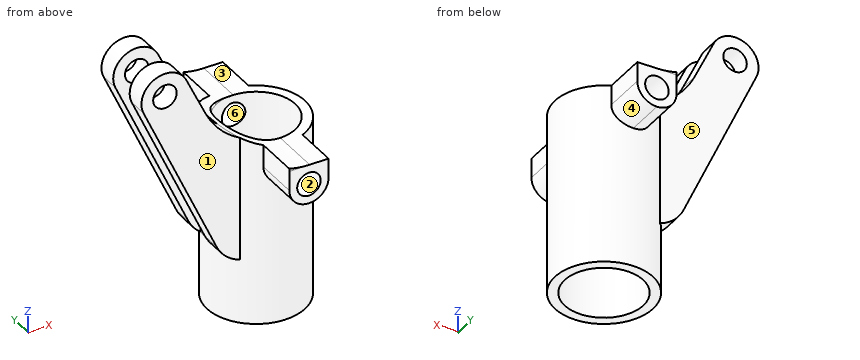
```python
from build123d import *

# Parameters (mm, degrees)
CROQUIS1_R                   = 6.25
CROQUIS1_R_2                 = 5
SALIENTE_EXTRUIR1_DEPTH      = 15
SALIENTE_EXTRUIR2_REACH      = 25.881
SALIENTE_EXTRUIR2_END_RADIUS = 6.25
CROQUIS2_W                   = 5
CROQUIS2_H                   = 5
SALIENTE_EXTRUIR3_REACH      = 29.755
SALIENTE_EXTRUIR3_END_RADIUS = 6.25
CROQUIS3_W                   = 5
CROQUIS3_H                   = 5
CORTAR_EXTRUIR1_REACH        = 29.755
CROQUIS4_R                   = 1.5
REDONDEO1_R                  = 2.5
CROQUIS5_R                   = 1.5
SALIENTE_EXTRUIR4_DEPTH      = 2.5
SALIENTE_EXTRUIR5_REACH      = 34.452
CROQUIS6_W                   = 15
CROQUIS6_H                   = 2.5
CROQUIS7_R                   = 1.5
SALIENTE_EXTRUIR6_DEPTH      = 2.5
SALIENTE_EXTRUIR7_REACH      = 34.452
SALIENTE_EXTRUIR7_END_RADIUS = 6.25
CROQUIS8_W                   = 15
CROQUIS8_H                   = 2.5
REDONDEO2_R                  = 5
REDONDEO4_R                  = 10
SALIENTE_EXTRUIR9_REACH      = 43.224
CROQUIS10_R                  = 6.25
CROQUIS10_R_2                = 5


# Some blends are built 0.0001 mm under size
with BuildPart() as part:
    # Croquis1 → Saliente-Extruir1 (new body)
    with BuildSketch(Plane.XY):
        Circle(CROQUIS1_R)
        Circle(CROQUIS1_R_2, mode=Mode.SUBTRACT)
    extrude(amount=SALIENTE_EXTRUIR1_DEPTH)

    # Saliente-Extruir2: up to this cylinder (the profile starts outside it)
    saliente_extruir2_end = Plane(origin=(0, 0, 12.5), z_dir=(0, 0, -1)) * Cylinder(SALIENTE_EXTRUIR2_END_RADIUS, 65.262, mode=Mode.PRIVATE)
    # Croquis2 → Saliente-Extruir2 (add, up to the surface)
    with BuildSketch(Plane(origin=(0, 11.25, 0), x_dir=(1, 0, 0), z_dir=(0, 1, 0)), mode=Mode.PRIVATE) as saliente_extruir2_sk1:
        with Locations((0, -12.5)):
            Rectangle(CROQUIS2_W, CROQUIS2_H)
    saliente_extruir2_tool1 = extrude(saliente_extruir2_sk1.sketch, amount=-SALIENTE_EXTRUIR2_REACH, mode=Mode.PRIVATE) - saliente_extruir2_end
    add(saliente_extruir2_tool1.solids().sort_by_distance((0, 11.25, 12.5))[0])

    # Saliente-Extruir3: up to this cylinder (the profile starts outside it)
    saliente_extruir3_end = Plane(origin=(0, 0, 12.5), z_dir=(0, 0, -1)) * Cylinder(SALIENTE_EXTRUIR3_END_RADIUS, 73.01, mode=Mode.PRIVATE)
    # Croquis3 → Saliente-Extruir3 (add, up to the surface)
    with BuildSketch(Plane(origin=(0, -11.25, 0), x_dir=(1, 0, 0), z_dir=(0, 1, 0)), mode=Mode.PRIVATE) as saliente_extruir3_sk1:
        with Locations((0, -12.5)):
            Rectangle(CROQUIS3_W, CROQUIS3_H)
    saliente_extruir3_tool1 = extrude(saliente_extruir3_sk1.sketch, amount=SALIENTE_EXTRUIR3_REACH, mode=Mode.PRIVATE) - saliente_extruir3_end
    add(saliente_extruir3_tool1.solids().sort_by_distance((0, -11.25, 12.5))[0])

    # Cortar-Extruir1: up to this face of the body (flat: up to its plane)
    cortar_extruir1_end = Plane(part.part.faces().sort_by_distance((0, -11.25, 12.5))[0])
    # Croquis4 → Cortar-Extruir1 (cut, up to the picked face)
    with BuildSketch(Plane(origin=(0, 11.25, 0), x_dir=(1, 0, 0), z_dir=(0, 1, 0)), mode=Mode.PRIVATE) as cortar_extruir1_sk1:
        with Locations(Location((0, -12.5, 0), (0, 0, 270))):
            Circle(CROQUIS4_R)
    cortar_extruir1_tool1 = split(extrude(cortar_extruir1_sk1.sketch, amount=-CORTAR_EXTRUIR1_REACH, mode=Mode.PRIVATE), bisect_by=cortar_extruir1_end, keep=Keep.BOTH, mode=Mode.PRIVATE)
    add(cortar_extruir1_tool1.solids().sort_by(Axis((0, 11.25, 12.5), (0, -1, 0)))[0], mode=Mode.SUBTRACT)

    # Redondeo1
    redondeo1_edges = [part.edges().sort_by_distance(p)[0] for p in [
        (-2.5, -8.489109809, 10),
        (2.5, -8.489109809, 10),
        (-2.5, 8.489109809, 10),
        (2.5, 8.489109809, 10),
    ]]
    fillet(redondeo1_edges, radius=REDONDEO1_R - 0.0001)  # a hair under: the kernel refuses the full size

    # Croquis6 → Saliente-Extruir5 (add, up to next)
    with BuildSketch(Plane(origin=(-6.25, 0, 0), x_dir=(0, 0, -1), z_dir=(1, 0, 0)), mode=Mode.PRIVATE) as saliente_extruir5_sk1:
        with Locations((-7.5, -3)):
            Rectangle(CROQUIS6_W, CROQUIS6_H)
    saliente_extruir5_tool1 = extrude(saliente_extruir5_sk1.sketch, amount=SALIENTE_EXTRUIR5_REACH, mode=Mode.PRIVATE) - part.part


with BuildPart() as body_2:
    # Croquis5 → Saliente-Extruir4 (new body)
    with BuildSketch(Plane(origin=(0, -4.25, 0), x_dir=(1, 0, 0), z_dir=(0, 1, 0))):
        with BuildLine():
            Line((-6.25, -15), (-11.445879417, -26.033157432))
            ThreePointArc((-11.445879417, -26.033157432), (-15.41753329, -27.478700895), (-16.893124871, -23.518112569))
            Line((-16.893124871, -23.518112569), (-6.25, 0))
            Line((-6.25, 0), (-6.25, -15))
        make_face()
        with Locations(Location((-14.159974768, -24.755, 0), (0, 0, 270))):
            Circle(CROQUIS5_R, mode=Mode.SUBTRACT)
    extrude(amount=SALIENTE_EXTRUIR4_DEPTH)


with BuildPart() as part_1:
    add(part.part)

    add(body_2.part)  # Saliente-Extruir5 merges body 2
    add(saliente_extruir5_tool1.solids().sort_by_distance((-6.25, -3, 7.5))[0])



with BuildPart() as body_2_2:
    # Croquis7 → Saliente-Extruir6 (new body)
    with BuildSketch(Plane(origin=(0, 4.25, 0), x_dir=(1, 0, 0), z_dir=(0, 1, 0))):
        with BuildLine():
            Line((-11.445879417, -26.033157432), (-6.25, -15))
            Line((-6.25, -15), (-6.25, 0))
            Line((-6.25, 0), (-16.893124871, -23.518112569))
            ThreePointArc((-16.893124871, -23.518112569), (-15.41753329, -27.478700895), (-11.445879417, -26.033157432))
        make_face()
        with Locations(Location((-14.159974768, -24.755, 0), (0, 0, 270))):
            Circle(CROQUIS7_R, mode=Mode.SUBTRACT)
    extrude(amount=-SALIENTE_EXTRUIR6_DEPTH)


with BuildPart() as part_2:
    add(part_1.part)

    add(body_2_2.part)  # Saliente-Extruir7 merges body 2 2
    # Saliente-Extruir7: up to this cylinder (the profile starts outside it)
    saliente_extruir7_end = Plane(origin=(0, 0, 7.5), z_dir=(0, 0, -1)) * Cylinder(SALIENTE_EXTRUIR7_END_RADIUS, 82.404, mode=Mode.PRIVATE)
    # Croquis8 → Saliente-Extruir7 (add, up to the surface)
    with BuildSketch(Plane(origin=(-6.25, 0, 0), x_dir=(0, 0, -1), z_dir=(1, 0, 0)), mode=Mode.PRIVATE) as saliente_extruir7_sk1:
        with Locations((-7.5, 3)):
            Rectangle(CROQUIS8_W, CROQUIS8_H)
    saliente_extruir7_tool1 = extrude(saliente_extruir7_sk1.sketch, amount=SALIENTE_EXTRUIR7_REACH, mode=Mode.PRIVATE) - saliente_extruir7_end
    add(saliente_extruir7_tool1.solids().sort_by_distance((-6.25, 3, 7.5))[0])

    # Redondeo2
    # the kernel refuses this fillet: 5 mm, written as the material it takes off along each edge
    with BuildSketch(Plane(origin=(-6.25, 12.313555344, 0), x_dir=(1, 0, 0), z_dir=(0, -1, 0))) as redondeo2_piece_1:
        with BuildLine():
            CenterArc((REDONDEO2_R * 0.645084427485, REDONDEO2_R), REDONDEO2_R, 204.349135832, 65.650864168)
            Line((-REDONDEO2_R * 0.265965606724, REDONDEO2_R * 0.587704189728), (0, 0))
            Line((0, 0), (REDONDEO2_R * 0.645084427485, 0))
        make_face()
    extrude(amount=18.627110687, mode=Mode.SUBTRACT)

    # Redondeo4
    # the kernel refuses this fillet: 10 mm, written as the material it adds along each edge
    with BuildSketch(Plane(origin=(-6.25, 20.110188614, 15), x_dir=(1, 0, 0), z_dir=(0, -1, 0))) as redondeo4_piece_1_section:
        with BuildLine():
            CenterArc((REDONDEO4_R * 0.634407544548, REDONDEO4_R), REDONDEO4_R, 205.2173, 64.7827)
            Line((-REDONDEO4_R * 0.27029090604, REDONDEO4_R * 0.573947522594), (0, 0))
            Line((0, 0), (REDONDEO4_R * 0.634407544548, 0))
        make_face()
    redondeo4_piece_1 = extrude(amount=34.220377227, mode=Mode.PRIVATE)
    redondeo4_piece_1 = split(redondeo4_piece_1, bisect_by=Plane(origin=(-2.5, 8.596165387, 15.10356988), z_dir=(1, 0, 0)), keep=Keep.TOP, mode=Mode.PRIVATE)
    redondeo4_piece_1 = split(redondeo4_piece_1, bisect_by=Plane(origin=(-1.866709216, -11.25, 15.10356988), z_dir=(0, 1, 0)), keep=Keep.TOP, mode=Mode.PRIVATE)
    redondeo4_piece_1 = split(redondeo4_piece_1, bisect_by=Plane(origin=(-1.866709216, 11.25, 15.10356988), z_dir=(0, -1, 0)), keep=Keep.TOP, mode=Mode.PRIVATE)
    redondeo4_piece_1 = redondeo4_piece_1 - Plane(origin=(0, 0, 15.10356988), x_dir=(1, 0, 0), z_dir=(0, 0, -1)) * Cylinder(5, 94, mode=Mode.PRIVATE)
    add(redondeo4_piece_1)
    with BuildSketch(Plane(origin=(-6.25, 4.25, 15), x_dir=(1, 0, 0), z_dir=(0, -1, 0))) as redondeo4_piece_2_section:
        with BuildLine():
            CenterArc((REDONDEO4_R * 0.634407544548, REDONDEO4_R), REDONDEO4_R, 205.2173, 64.7827)
            Line((-REDONDEO4_R * 0.27029090604, REDONDEO4_R * 0.573947522594), (0, 0))
            Line((0, 0), (REDONDEO4_R * 0.634407544548, 0))
        make_face()
    redondeo4_piece_2 = extrude(amount=2.5, mode=Mode.PRIVATE)
    redondeo4_piece_2 = redondeo4_piece_2 - Plane(origin=(0, 0, 16.752062652), x_dir=(1, 0, 0), z_dir=(0, 0, -1)) * Cylinder(5, 31, mode=Mode.PRIVATE)
    add(redondeo4_piece_2)
    with BuildSketch(Plane(origin=(-6.25, 20.110188614, 15), x_dir=(1, 0, 0), z_dir=(0, -1, 0))) as redondeo4_piece_3_section:
        with BuildLine():
            CenterArc((REDONDEO4_R * 0.634407544548, REDONDEO4_R), REDONDEO4_R, 205.2173, 64.7827)
            Line((-REDONDEO4_R * 0.27029090604, REDONDEO4_R * 0.573947522594), (0, 0))
            Line((0, 0), (REDONDEO4_R * 0.634407544548, 0))
        make_face()
    redondeo4_piece_3 = extrude(amount=34.220377227, mode=Mode.PRIVATE)
    redondeo4_piece_3 = redondeo4_piece_3 & Plane(origin=(0, 0, 15.324058302), x_dir=(1, 0, 0), z_dir=(0, 0, -1)) * Cylinder(6.25, 94, mode=Mode.PRIVATE)
    redondeo4_piece_3 = redondeo4_piece_3 - Plane(origin=(0, 0, 15.324058302), x_dir=(1, 0, 0), z_dir=(0, 0, -1)) * Cylinder(5, 94, mode=Mode.PRIVATE)
    add(redondeo4_piece_3)
    with BuildSketch(Plane(origin=(-6.25, 20.110188614, 15), x_dir=(1, 0, 0), z_dir=(0, -1, 0))) as redondeo4_piece_4_section:
        with BuildLine():
            CenterArc((REDONDEO4_R * 0.634407544548, REDONDEO4_R), REDONDEO4_R, 205.2173, 64.7827)
            Line((-REDONDEO4_R * 0.27029090604, REDONDEO4_R * 0.573947522594), (0, 0))
            Line((0, 0), (REDONDEO4_R * 0.634407544548, 0))
        make_face()
    redondeo4_piece_4 = extrude(amount=34.220377227, mode=Mode.PRIVATE)
    redondeo4_piece_4 = split(redondeo4_piece_4, bisect_by=Plane(origin=(-6.508076771, -4.25, 16.752062651), z_dir=(0, 1, 0)), keep=Keep.TOP, mode=Mode.PRIVATE)
    redondeo4_piece_4 = split(redondeo4_piece_4, bisect_by=Plane(origin=(-6.508076771, -1.75, 16.752062651), z_dir=(0, -1, 0)), keep=Keep.TOP, mode=Mode.PRIVATE)
    redondeo4_piece_4 = redondeo4_piece_4 - Plane(origin=(0, 0, 16.752062651), x_dir=(1, 0, 0), z_dir=(0, 0, -1)) * Cylinder(5, 94, mode=Mode.PRIVATE)
    add(redondeo4_piece_4)

    # Croquis10 → Saliente-Extruir9 (add, up to next)
    with BuildSketch(Plane(origin=(0, 0, -8), x_dir=(-1, 0, 0), z_dir=(0, 0, -1)), mode=Mode.PRIVATE) as saliente_extruir9_sk1:
        Circle(CROQUIS10_R)
        Circle(CROQUIS10_R_2, mode=Mode.SUBTRACT)
    saliente_extruir9_tool1 = extrude(saliente_extruir9_sk1.sketch, amount=-SALIENTE_EXTRUIR9_REACH, mode=Mode.PRIVATE) - part_2.part
    add(saliente_extruir9_tool1.solids().sort_by_distance((6.073223, 0, -8))[0])


solid = part_2.part
```
Geometry check sheet. Reference: the model listing, model coordinates, mm. Face numbers are marked on the shaded views. A direction names the side the tool comes from. Give positions to 0.01 mm unless a question says otherwise; leave off trailing zeros. Order: outer loops, then holes, each group sorted by start corner. A loop starts at its lowest first (then second) coordinate and runs counter-clockwise, first axis right, second up. Notation, with made-up numbers: (83, -12.75) - (139, -12.75) arc R20 cw to (139, 5.25) - close; hole circle Ø2 at (-12.75, 26). An arc over 180 degrees is marked (long way). Answer in a Markdown table with one row per item. Add a question column.
Q1. Cross-section at D-D, the plane z = 6. Enter the section's corners in (x, y).
Q2. Material ranges on probe 1 along X at (y, z) = (0, 8.75); probe 2 along Z at (x, y) = (0, 9); probe 3 along X at (y, z) = (-5.75, 12.5), recorded low to high. Write a range as from..to.
Q3. Mould release check, pull along X, two halves, no side actions. Record for the marked faces 4, 5 and 6: pulls with the +X half, pulls with the -X half, needs draft (parallel to the pull), parting line crosses it, or undercut.
Q4. Cross-section at B-B, the plane x = 2. Enter the section's corners in (y, z).
Q5. Tool access check on the marked faces 1, 2 and 3. Record the directions out of +Z, -Z, +X, -X, +Y, -Y that give a thin tool (end or side, any length) a straight path to the whole face; none if there is none.
Q6. Gauge pin test, flat ends, axial feed: pin 1 (6.5 mm diameter, centred on x = -9, z = 8, fed in from +Y); pin 2 (5 mm diameter, centred on y = -1, z = 13.5, fed in from +X); pin 3 (10 mm diameter, centred on x = -4, z = 6, fed in from -Y); pin 4 (6 mm diameter, centred on x = 0, y = 0, fed in from +Z). Record the tip position at first contact, or that the pin passes through.
Q7. Cross-section at C-C, the plane y = 0. Enter the section's corners in (x, z).
Check values:
| question | item | result |
|---|---|---|
| 1 | outline | (-8.97, -4.25) - (-4.58, -4.25) arc R6.25 ccw (long way) to (-4.58, 4.25) - (-8.97, 4.25) - (-8.97, 1.75) - (-6, 1.75) arc R6.25 ccw to (-6, -1.75) - (-8.97, -1.75) - close; hole circle Ø10 at (0, 0) |
| 2 | probe 1 | x = -6.25..-5, 5..6.25 |
| 2 | probe 2 | z = 10..11, 14..15 |
| 2 | probe 3 | x = -2.5..-1.5, 1.5..2.5 |
| 3 | face 4 | pulls with the +X half |
| 3 | face 5 | needs draft |
| 3 | face 6 | undercut |
| 4 | outline | (-11.25, 11) - (-5.92, 11) - (-5.92, -8) - (-4.58, -8) - (-4.58, 15) - (-11.25, 15) - close; (4.58, -8) - (5.92, -8) - (5.92, 11) - (11.25, 11) - (11.25, 15) - (4.58, 15) - close |
| 5 | face 1 | +Z, -Z, -X, -Y |
| 5 | face 2 | +Y, -Y |
| 5 | face 3 | +Z, +X, +Y, -Y |
| 6 | pin 1 | stops at y = 4.25 |
| 6 | pin 2 | stops at x = 6.25 |
| 6 | pin 3 | stops at y = -6.25 |
| 6 | pin 4 | passes through |
| 7 | outline | (-6.25, -8) - (-5, -8) - (-5, 16.39) arc R10 cw to (-6.25, 17.27) - close; (5, -8) - (6.25, -8) - (6.25, 15) - (5, 15) - close |
